The model under review builds one solid part; all positions refer to its coordinate system, in mm. A direction names the side the tool comes from. Coordinates: 2 decimals unless noted, no trailing zeros. Order: outer loops, then holes, each group sorted by start corner. A loop starts at its lowest first (then second) coordinate and runs counter-clockwise, first axis right, second up. Notation, with made-up numbers: M 43,28.5 L 88,28.5 A25 ccw 88,61.5 Z; hole C 37.25,6.25 d1. An arc over 180 degrees is marked long. One line per item, written item: value.
```python
from build123d import *

# Parameters (mm, degrees)
F1_DEPTH = 4
F2_R     = 2
F3_DEPTH = 4
F4_W     = 53
F4_H     = 53
F5_DEPTH = 2
F6_R     = 1


with BuildPart() as f1:
    # F0 (on Top) → F1 (new body)
    with BuildSketch(Plane.XY):
        with BuildLine():
            ThreePointArc((-28.5, 24), (-25.6715728753, 25.1715728753), (-24.5, 28))
            Line((-24.5, 28), (-28.5, 28))
            Line((-28.5, 28), (-28.5, 24))
        make_face()
        with BuildLine():
            Line((-28.5, 28), (-24.5, 28))
            ThreePointArc((-24.5, 28), (-31.3284271247, 30.8284271247), (-28.5, 24))
            Line((-28.5, 24), (-28.5, 28))
        make_face()
        with BuildLine():
            Line((24.5, 28), (-24.5, 28))
            ThreePointArc((-24.5, 28), (-25.6715728753, 25.1715728753), (-28.5, 24))
            Line((-28.5, 24), (-28.5, -24))
            ThreePointArc((-28.5, -24), (-25.6715728753, -25.1715728753), (-24.5, -28))
            Line((-24.5, -28), (24.5, -28))
            ThreePointArc((24.5, -28), (25.6715728753, -25.1715728753), (28.5, -24))
            Line((28.5, -24), (28.5, 24))
            ThreePointArc((28.5, 24), (25.6715728753, 25.1715728753), (24.5, 28))
        make_face()
        with BuildLine():
            ThreePointArc((32.5, 28), (28.5, 32), (24.5, 28))
            Line((24.5, 28), (28.5, 28))
            Line((28.5, 28), (28.5, 24))
            ThreePointArc((28.5, 24), (31.3284271247, 25.1715728753), (32.5, 28))
        make_face()
        with BuildLine():
            Line((28.5, 28), (24.5, 28))
            ThreePointArc((24.5, 28), (25.6715728753, 25.1715728753), (28.5, 24))
            Line((28.5, 24), (28.5, 28))
        make_face()
        with BuildLine():
            ThreePointArc((-24.5, -28), (-25.6715728753, -25.1715728753), (-28.5, -24))
            Line((-28.5, -24), (-28.5, -28))
            Line((-28.5, -28), (-24.5, -28))
        make_face()
        with BuildLine():
            Line((-28.5, -28), (-28.5, -24))
            ThreePointArc((-28.5, -24), (-31.3284271247, -30.8284271247), (-24.5, -28))
            Line((-24.5, -28), (-28.5, -28))
        make_face()
        with BuildLine():
            ThreePointArc((32.5, -28), (31.3284271247, -25.1715728753), (28.5, -24))
            Line((28.5, -24), (28.5, -28))
            Line((28.5, -28), (24.5, -28))
            ThreePointArc((24.5, -28), (28.5, -32), (32.5, -28))
        make_face()
        with BuildLine():
            Line((28.5, -28), (28.5, -24))
            ThreePointArc((28.5, -24), (25.6715728753, -25.1715728753), (24.5, -28))
            Line((24.5, -28), (28.5, -28))
        make_face()
    extrude(amount=F1_DEPTH)

    # F2 (on face) → F3 (cut, through all)
    with BuildSketch(Plane.XY.offset(4)):
        with Locations((-28.5, 28)):
            Circle(F2_R)
        with Locations((28.5, 28)):
            Circle(F2_R)
        with Locations((28.5, -28)):
            Circle(F2_R)
        with Locations((-28.5, -28)):
            Circle(F2_R)
    extrude(amount=-F3_DEPTH, mode=Mode.SUBTRACT)

    # F4 (on face) → F5 (cut)
    with BuildSketch(Plane.XY.offset(4)):
        Rectangle(F4_W, F4_H)
    extrude(amount=-F5_DEPTH, mode=Mode.SUBTRACT)

    # F6
    f6_edges = [f1.edges().sort_by_distance(p)[0] for p in [
        (-26.5, 26.5, 3),
        (26.5, 26.5, 3),
        (26.5, -26.5, 3),
        (-26.5, -26.5, 3),
    ]]
    fillet(f6_edges, radius=F6_R)


solid = f1.part
```
(1) For L1, parallel to Y at x = 17.5, z = 3.15; L2, parallel to X at y = -18.5, z = 2.6; L3, parallel to X at y = -29, z = 1.7, list the stretches that pass through material, from the lowest coordinate up.
Geometry results:
L1: y = -28 to -26.5, 26.5 to 28
L2: x = -28.5 to -26.5, 26.5 to 28.5
L3: x = -32.37 to -30.23, -26.77 to -24.63, 24.63 to 26.77, 30.23 to 32.37
(2) Tool access review of faces 1 (the flat face through (-28.5, 0, 2)), 2 (the flat face through (26.5, 0, 3)), 3 (the flat face through (0, 28, 2)): name each direction out of +Z, -Z, +X, -X, +Y, -Y from which nothing blocks a thin tool from reaching the whole face with its end or side.
Geometry results:
face 1: +Z, -Z, -X
face 2: +Z
face 3: +Z, -Z, +Y
(3) Insertion check: pin 1 Ø0.6 at (x, z) = (8, 3) entering from +Y; pin 2 Ø2 at (y, z) = (12.5, 1.5) entering from +X; pin 3 Ø8 at (x, y) = (12, -15) entering from +Z; pin 4 Ø3.5 at (x, y) = (28.5, -28) entering from -Z. Each pin has a flat end and moves straight along its axis. Give the tip position at first contact, or say it passes through.
Geometry results:
pin 1: stops at y = 28
pin 2: stops at x = 28.5
pin 3: stops at z = 2
pin 4: passes through
(4) We need section A-A, the plane x = -9. State the section outline as (y, z) points.
Geometry results:
outline: M -28,0 L 28,0 L 28,4 L 26.5,4 L 26.5,2 L -26.5,2 L -26.5,4 L -28,4 Z
(5) Mouldability with a two-part tool opening along X and no side actions: class faces 4 (the flat face through (-27, -2, 4)), 5 (the flat face through (28.5, 0, 2)), 6 (the flat face through (0, -28, 2)), 7 (the cylindrical face through (29.423, -29.774, 2.028)) as +X half, -X half, draft (parallel to the pull), parting line (faces both ways), or undercut.
Geometry results:
face 4: draft
face 5: +X half
face 6: undercut
face 7: undercut
(6) We need section B-B, the plane y = -16. State the section outline as (x, z) points.
Geometry results:
outline: M -28.5,0 L 28.5,0 L 28.5,4 L 26.5,4 L 26.5,2 L -26.5,2 L -26.5,4 L -28.5,4 Z
